Could you check a few things on this model? Use its own coordinates, in mm. A direction names the side the tool comes from. Coordinates: 2 decimals unless noted, no trailing zeros. Write each loop counter-clockwise with the first axis right and the second up, starting at its lowest first coordinate (ties: lowest second). Pieces come first, ordered by that corner, then holes. Notation, with made-up numbers: M -16,-4 L 14,-4 A26 ccw 14,32 Z; hole C 28,43.25 d10. An arc over 180 degrees is marked long. Write item = value, one per line.
```python
from build123d import *

# Parameters (mm, degrees)
SKETCH1_R           = 1.75
BOSS_EXTRUDE1_DEPTH = 15
SKETCH2_R           = 2.25
SKETCH2_W           = 20
SKETCH2_H           = 5
CUT_EXTRUDE1_DEPTH  = 15


with BuildPart() as part:
    # Sketch1 → Boss-Extrude1 (new body)
    with BuildSketch(Plane.XY):
        with BuildLine():
            Line((50, 57.5), (50, 65))
            Line((50, 65), (-50, 65))
            Line((-50, 65), (-50, 57.5))
            Line((-50, 57.5), (-45, 57.5))
            ThreePointArc((-45, 57.5), (-44.172482646, 57.640929202), (-43.438262381, 58.047827976))
            ThreePointArc((-43.438262381, 58.047827976), (-41.351700501, 59.204183244), (-39, 59.604686356))
            Line((-39, 59.604686356), (39, 59.604686356))
            ThreePointArc((39, 59.604686356), (41.351700501, 59.204183244), (43.438262381, 58.047827976))
            ThreePointArc((43.438262381, 58.047827976), (44.172482646, 57.640929202), (45, 57.5))
            Line((45, 57.5), (50, 57.5))
        make_face()
        with Locations((45, 60)):
            Circle(SKETCH1_R, mode=Mode.SUBTRACT)
        with Locations(Location((-45, 60, 0), (0, 0, 180))):
            Circle(SKETCH1_R, mode=Mode.SUBTRACT)
    extrude(amount=BOSS_EXTRUDE1_DEPTH)

    # Sketch2 → Cut-Extrude1 (cut)
    with BuildSketch(Plane(origin=(0, 65, 0), x_dir=(1, 0, 0), z_dir=(0, 1, 0))):
        with Locations(Location((35, -7.5, 0), (0, 0, 270))):
            Circle(SKETCH2_R)
        with Locations(Location((-35, -7.5, 0), (0, 0, 270))):
            Circle(SKETCH2_R)
        with Locations((0, -2.5)):
            Rectangle(SKETCH2_W, SKETCH2_H)
    extrude(amount=-CUT_EXTRUDE1_DEPTH, mode=Mode.SUBTRACT)


solid = part.part
```
Item 1: Imagine slicing it at C-C (z = 2). Write out the boundary of the cut face in (x, y).
Numbers:
outline = M -50,57.5 L -45,57.5 A2.5 ccw -43.44,58.05 A7.1 cw -39,59.6 L -10,59.6 L -10,65 L -50,65 Z; M 10,59.6 L 39,59.6 A7.1 cw 43.44,58.05 A2.5 ccw 45,57.5 L 50,57.5 L 50,65 L 10,65 Z; hole C -45,60 d3.5; hole C 45,60 d3.5
Item 2: Imagine slicing it at D-D (y = 63.75). Write out the boundary of the cut face in (x, z), and give its area (3 significant figures).
Numbers:
outline = M -50,0 L -10,0 L -10,5 L 10,5 L 10,0 L 50,0 L 50,15 L -50,15 Z; hole C -35,7.5 d4.5; hole C 35,7.5 d4.5
area = 1,370 mm²
Item 3: For faces 4 (the face through (10, 62, 3)), 5 (the face through (30, 62, 0)), 6 (the face through (-41.383, 59.193, 7.395)), which set-ups out of +Z, -Z, +X, -X, +Y, -Y let a thin tool reach every point of the face, with its end or its side?
Numbers:
face_4 = -Z, +Y, -Y
face_5 = -Z, +X, -X, +Y, -Y
face_6 = +Z, -Z, -Y
Item 4: Imagine slicing it at A-A (z = 7.5). Write out the boundary of the cut face in (x, y), and give its area (3 significant figures).
Numbers:
outline = M -50,57.5 L -45,57.5 A2.5 ccw -43.44,58.05 A7.1 cw -39,59.6 L -37.25,59.6 L -37.25,65 L -50,65 Z; M -32.75,59.6 L 32.75,59.6 L 32.75,65 L -32.75,65 Z; M 37.25,59.6 L 39,59.6 A7.1 cw 43.44,58.05 A2.5 ccw 45,57.5 L 50,57.5 L 50,65 L 37.25,65 Z; hole C -45,60 d3.5; hole C 45,60 d3.5
area = 503 mm²
Item 5: If we mould it in two halves opening along Y, with no side actions, what happens to faces 1 (the face through (-48, 57.5, 7)), 2 (the face through (46.617, 59.33, 7.395)), 3 (the face through (-1, 62, 15))? For each: pulls with the +Y half, pulls with the -Y half, needs draft (parallel to the pull), parting line crosses it, or undercut.
Numbers:
face_1 = pulls with the -Y half
face_2 = undercut
face_3 = needs draft
Item 6: I'm going to push a flat-ended pin straight in: P1, Ø5, axis at x = 35, z = 7.5, coming from the -Y side. Where does the tip first touch, or does it pass through?
Numbers:
P1 = 59.6
Item 7: Imagine slicing it at B-B (x = 35). Write out the boundary of the cut face in (y, z), and give its area (3 significant figures).
Numbers:
outline = M 59.6,0 L 65,0 L 65,5.25 L 59.6,5.25 Z; M 59.6,9.75 L 65,9.75 L 65,15 L 59.6,15 Z
area = 56.7 mm²
Item 8: If I drill on line 1 along X through (y, z) = (62.5, 7.5); line 2 along Y through (x, z) = (-45, 6.75); line 3 along X through (y, z) = (60.8, 7.5), over which ranges is the centre line in solid material (lowest first)?
Numbers:
line_1 = -50 to -37.25, -32.75 to 32.75, 37.25 to 50
line_2 = 57.5 to 58.25, 61.75 to 65
line_3 = -50 to -46.56, -43.44 to -37.25, -32.75 to 32.75, 37.25 to 43.44, 46.56 to 50
